Here's how the part is built. I have some questions about the finished solid (model axes, mm). Face numbers are marked on the shaded views. A direction names the side the tool comes from. Coordinates: 2 decimals unless noted, no trailing zeros. Write each loop counter-clockwise with the first axis right and the second up, starting at its lowest first coordinate (ties: lowest second). Pieces come first, ordered by that corner, then holes. Notation, with made-up numbers: M 58.25,-39.75 L 113.25,-39.75 A36 ccw 113.25,-3.75 Z; hole C 8.5,66 d3. An arc over 180 degrees is marked long. Write each question's results on one line, items separated by ' | '. Start each with the question number.
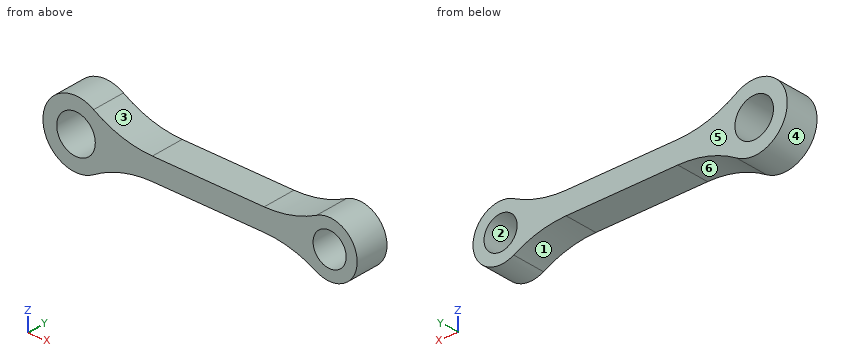
from build123d import *

# Parameters (mm, degrees)
SKETCH1_R           = 1.75
SKETCH1_R_2         = 1.5
BOSS_EXTRUDE1_DEPTH = 3


with BuildPart() as part:
    # Sketch1 → Boss-Extrude1 (new body)
    with BuildSketch(Plane(origin=(0, 0, 0), x_dir=(1, 0, 0), z_dir=(0, 1, 0))):
        with BuildLine():
            Line((6.92820323, 1), (17.062828956, 1))
            ThreePointArc((17.062828956, 1), (19.512318699, 1.304640285), (21.812565791, 2.2))
            ThreePointArc((21.812565791, 2.2), (25.5, 0), (21.812565791, -2.2))
            ThreePointArc((21.812565791, -2.2), (19.512318699, -1.304640285), (17.062828956, -1))
            Line((17.062828956, -1), (6.92820323, -1))
            ThreePointArc((6.92820323, -1), (4.154702249, -1.392310772), (1.59881613, -2.538461538))
            ThreePointArc((1.59881613, -2.538461538), (-3, 0), (1.59881613, 2.538461538))
            ThreePointArc((1.59881613, 2.538461538), (4.154702249, 1.392310772), (6.92820323, 1))
        make_face()
        Circle(SKETCH1_R, mode=Mode.SUBTRACT)
        with Locations((23, 0)):
            Circle(SKETCH1_R_2, mode=Mode.SUBTRACT)
    extrude(amount=BOSS_EXTRUDE1_DEPTH)


solid = part.part
1) For pin 1 Ø1.5 at (x, y) = (14, 1.5) entering from +Z; pin 2 Ø1.5 at (y, z) = (1, 2) entering from +X, each with a flat end and sliding along its axis, tell me the tip position at first contact or that it passes through.
2) We'd pull the mould along X, two halves only. Please class the marked faces 4, 5 and 6: pulls with the +X half, pulls with the -X half, needs draft (parallel to the pull), parting line crosses it, or undercut.
3) I want a section at D-D, the plane x = 23. Write out the boundary of the cut face in (y, z).
4) I want a section at A-A, the plane z = 0. Write out the boundary of the cut face in (x, y), then the cut area to 3 significant figures.
5) I want a section at B-B, the plane x = 0. Write out the boundary of the cut face in (y, z), then the cut area to 3 significant figures.
6) I want a section at C-C, the plane y = 1.1. Write out the boundary of the cut face in (x, z), then the cut area to 3 significant figures.
7) For the marked faces 1, 2 and 3, which set-ups out of +Z, -Z, +X, -X, +Y, -Y let a thin tool reach every point of the face, with its end or its side?
8) Please list where these lines run through material, in increasing order: line 1 (Z direction, x = 0, y = 2.6); line 2 (X direction, y = 2.25, z = -0.75); line 3 (Z direction, x = 17.25, y = 2.7). Write a range as [from, to].
Output:
1) pin 1: stops at z = 1 | pin 2: stops at x = 25.17
2) face 4: parting line crosses it | face 5: needs draft | face 6: undercut
3) outline: M 0,-2.5 L 3,-2.5 L 3,-1.5 L 0,-1.5 Z; M 0,1.5 L 3,1.5 L 3,2.5 L 0,2.5 Z
4) outline: M -3,0 L -1.75,0 L -1.75,3 L -3,3 Z; M 1.75,0 L 21.5,0 L 21.5,3 L 1.75,3 Z; M 24.5,0 L 25.5,0 L 25.5,3 L 24.5,3 Z | area: 66.0 mm2
5) outline: M 0,-3 L 3,-3 L 3,-1.75 L 0,-1.75 Z; M 0,1.75 L 3,1.75 L 3,3 L 0,3 Z | area: 7.50 mm2
6) outline: M 1.6,-2.54 A10 cw 6.93,-1 L 17.06,-1 A10 cw 21.81,-2.2 A2.5 ccw long 21.81,2.2 A10 cw 17.06,1 L 6.93,1 A10 cw 1.6,2.54 A3 ccw long Z; hole C 0,0 d3.5; hole C 23,0 d3 | area: 71.5 mm2
7) face 1: -Z, +Y, -Y | face 2: +Y, -Y | face 3: +Z, +Y, -Y
8) line 1: z = [-3, -1.75], [1.75, 3] | line 2: x = [-2.9, -1.58], [1.58, 21.7], [24.3, 25.38] | line 3: z = [-1, 1]
